Solid Edge part; units mm, degrees
sketch "Sketch1" plane through (0, 0, 0) normal (0, 0, 1) x (1, 0, 0)
  line L0 (47.5, -17.5) -> (-47.5, -17.5)
  line L1 (-47.5, -17.5) -> (-47.5, 17.5)
  line L2 (-47.5, 17.5) -> (47.5, 17.5)
  line L3 (47.5, 17.5) -> (47.5, -17.5)
  dimension "D1" = 47.5
  dimension "D2" = 47.5
extrude "Protrusion1" add sketch "Sketch1" along normal blind 27
sketch "Sketch2" plane through (0, 0, 27) normal (0, 0, 1) x (1, 0, 0)
  line L0 (3.77, 15) -> (3.77, 17)
  line L1 (3.77, 17) -> (30.77, 17)
  line L2 (30.77, 17) -> (30.77, 8)
  line L3 (36.5, 8) -> (30.77, 8)
  line L4 (36.5, 9.25) -> (36.5, 8)
  line L5 (37.5, 9.25) -> (36.5, 9.25)
  line L6 (37.5, 10.5) -> (37.5, 9.25)
  line L7 (42.5, 10.5) -> (37.5, 10.5)
  line L8 (42.5, 9.25) -> (42.5, 10.5)
  line L9 (42.5, 9.25) -> (43.5, 9.25)
  line L10 (43.5, 9.25) -> (43.5, 8)
  line L11 (43.5, 8) -> (47.5, 8)
  line L12 (47.5, 8) -> (47.5, 0)
  line L13 (-47.5, 0) -> (-47.5, 8)
  line L14 (-43.23, 8) -> (-47.5, 8)
  line L15 (-43.23, 8) -> (-43.23, 9.25)
  line L16 (-43.23, 9.25) -> (-42.23, 9.25)
  line L17 (-42.23, 9.25) -> (-42.23, 10.5)
  line L18 (-42.23, 10.5) -> (-37.23, 10.5)
  line L19 (-37.23, 10.5) -> (-37.23, 9.25)
  line L20 (-37.23, 9.25) -> (-36.23, 9.25)
  line L21 (-36.23, 9.25) -> (-36.23, 8)
  line L22 (-21.23, 8) -> (-36.23, 8)
  line L23 (-21.23, 8) -> (-21.23, 15)
  line L24 (-21.23, 15) -> (3.77, 15)
  dimension "D1" = 3.77
revolve "RevolvedCutout1" cut sketch "Sketch2" angle 360 about axis through (47.5, 0, 27) along (-1, 0, 0)
sketch "Sketch3" plane through (0, -17.5, 13.5) normal (0, -1, 0) x (1, 0, 0)
  line L0 (3.77, 5) -> (30.77, 5)
  line L1 (30.77, 5) -> (30.77, 13.5)
  line L2 (30.77, 13.5) -> (3.77, 13.5)
  line L3 (3.77, 13.5) -> (3.77, 5)
extrude "Extrusionsausschnitt_1" cut sketch "Sketch3" against normal blind 7.5
sketch "Sketch4" plane through (17.27, -16.1112, 18.5) normal (0, 0, 1) x (1, 0, 0)
  line L0 (-13.5, 6.1112) -> (13.5, 6.1112)
  line L1 (-13.5, -1.3888) -> (-13.5, 6.1112)
  line L2 (13.5, -1.3888) -> (-13.5, -1.3888)
  line L3 (14.996, -1.3888) -> (13.5, -1.3888)
  line L4 (14.996, 6.1112) -> (14.996, -1.3888)
  line L5 (13.5, 6.1112) -> (14.996, 6.1112)
  dimension "D1" = 13.5
  dimension "D2" = 13.5
extrude "Extrusionsausschnitt_2" cut sketch "Sketch4" along normal mid plane 100
hole "Bohrung_1" at (-25.73, 13.5, 27) direction (0, 0, -1) diameter 2.459 depth 12
hole "Hole1" at (39.883, -13.5, 27) direction (0, 0, -1) diameter 2.459 depth 12
hole "Hole2" at (-25.73, -13.5, 27) direction (0, 0, -1) diameter 2.459 depth 12
hole "Hole3" at (-43, -13.5, 27) direction (0, 0, -1) diameter 2.459 depth 12
hole "Hole4" at (-43, 13.5, 27) direction (0, 0, -1) diameter 2.459 depth 12
hole "Hole5" at (44, 13.5, 27) direction (0, 0, -1) diameter 2.459 depth 12
hole "Bohrung_8" at (-33.23, -13.5, 0) direction (0, 0, 1) diameter 4.134 depth 16
hole "Hole6" at (39.88, 13.5, 0) direction (0, 0, 1) diameter 4.134 depth 16
hole "Hole7" at (39.883, -13.5, 0) direction (0, 0, 1) diameter 4.134 depth 16
hole "Hole8" at (-33.23, 13.5, 0) direction (0, 0, 1) diameter 4.134 depth 16
properties part number "32" material "Polykarbonat"
Input: part model. Units: mm. Frame: model coordinates. A direction names the side the tool comes from. Give positions to 0.01 mm unless a question says otherwise; leave off trailing zeros. Write each loop counter-clockwise with the first axis right and the second up, starting at its lowest first coordinate (ties: lowest second). Pieces come first, ordered by that corner, then holes. Notation, with made-up numbers: M 60.25,42.25 L 93.25,42.25 A14 ccw 93.25,60.25 Z; hole C -39,3.25 d9. An arc over 180 degrees is marked long. Write item = value, one per line. Start each with the question number.
1) Draft query along X for faces 1 (the cylindrical face through (17.459, 7.479, 11.734)), 2 (the flat face through (43.5, 0, 18.6)), 3 (the flat face through (-47.5, 0, 13)), 4 (the flat face through (-1, 17.5, 13)). Return one class per face: +X half, -X half, draft (parallel to the pull), parting line (faces both ways), or undercut.
2) Cut plane B-B on z = 4.25. Return the cut outline in (x, y), then the cut area to 3 significant figures.
3) Reachability of faces 5 (the flat face through (32.266, -14, 13)), 6 (the cylindrical face through (-35.28, -13.77, 8.11)), 7 (the flat face through (-21.23, 0, 18)) from +Z, -Z, +X, -X, +Y, -Y: full face, straight path, thin tool, end or side. Return the list, or none.
4) Cut plane D-D on y = 0. Return the cut outline in (x, z).
5) First-contact query: pin 1 Ø3 at (x, y) = (-25.73, 13.5) entering from -Z; pin 2 Ø2 at (y, z) = (-3.5, 23) entering from -X; pin 3 Ø10 at (x, y) = (-10, -5) entering from +Z; pin 4 Ø3.5 at (x, y) = (-33.23, -13.5) entering from -Z. Flat tips, straight axial feed; report the tip coordinate or a pass-through.
6) Cut plane A-A on y = -13.5. Count the separate pieces of the cut face and the enclosed holes in it, then the cut area to 3 significant figures.
7) Material intervals for line 1 along X through (y, z) = (-7, 20.5); line 2 along X through (y, z) = (13.5, 6.75); line 3 along Y through (x, z) = (-33.23, 9), sorted ascending. Write a range as [from, to].
8) Cut plane C-C on x = -25.73. Return the cut outline in (y, z).
Solved:
q1.face_1 = undercut
q1.face_2 = undercut
q1.face_3 = -X half
q1.face_4 = draft
q2.outline = M -47.5,-17.5 L 3.77,-17.5 L 3.77,-10 L 32.27,-10 L 32.27,-17.5 L 47.5,-17.5 L 47.5,17.5 L -47.5,17.5 Z; hole C -33.23,-13.5 d4.13; hole C -33.23,13.5 d4.13; hole C 39.88,13.5 d4.13; hole C 39.88,-13.5 d4.13
q2.area = 3,060 mm2
q3.face_5 = +Z, -Z, -Y
q3.face_6 = -Z
q3.face_7 = +Z
q4.outline = M -47.5,0 L 47.5,0 L 47.5,19 L 43.5,19 L 43.5,17.75 L 42.5,17.75 L 42.5,16.5 L 37.5,16.5 L 37.5,17.75 L 36.5,17.75 L 36.5,19 L 30.77,19 L 30.77,10 L 3.77,10 L 3.77,12 L -21.23,12 L -21.23,19 L -36.23,19 L -36.23,17.75 L -37.23,17.75 L -37.23,16.5 L -42.23,16.5 L -42.23,17.75 L -43.23,17.75 L -43.23,19 L -47.5,19 Z
q5.pin_1 = 0
q5.pin_2 = through
q5.pin_3 = 15.82
q5.pin_4 = 16
q6.separate_pieces = 3
q6.enclosed_holes = 0
q6.area = 1,410 mm2
q7.line_1 = [-47.5, -42.23], [-37.23, -21.23], [30.77, 37.5], [42.5, 47.5]
q7.line_2 = [-47.5, -35.3], [-31.16, 37.81], [41.95, 47.5]
q7.line_3 = [-17.5, -15.57], [-11.43, 11.43], [15.57, 17.5]
q8.outline = M -17.5,0 L 17.5,0 L 17.5,27 L 14.73,27 L 14.73,15 L 12.27,15 L 12.27,27 L 8,27 A8 cw -8,27 L -12.27,27 L -12.27,15 L -14.73,15 L -14.73,27 L -17.5,27 Z
